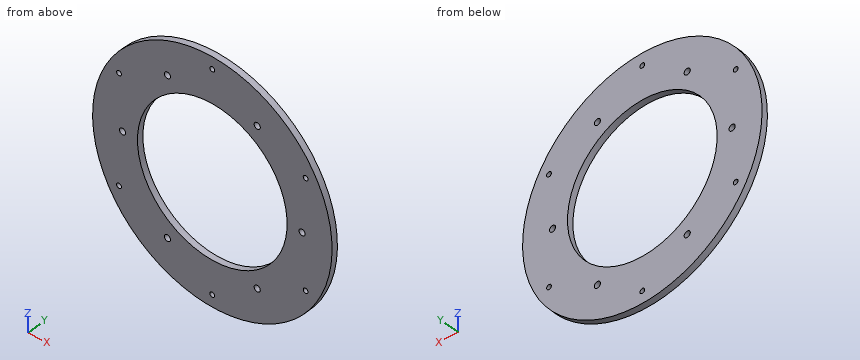
from build123d import *

# Parameters (mm, degrees)
SKETCH_1_R      = 80
SKETCH_1_R_2    = 50
SKETCH_1_R_3    = 2.05
EXTRUDE_1_DEPTH = 4
EXTRUDE_START   = -4
SKETCH_2_R      = 2.05
SKETCH_2_R_2    = 1.6
EXTRUDE_2_DEPTH = 4


with BuildPart() as part:
    # 草图1 → 凸台-拉伸1 (new body)
    with BuildSketch(Plane(origin=(0, 0, 0), x_dir=(1, 0, 0), z_dir=(0, 1, 0))):
        with Locations(Location((0, 0, 0), (0, 0, 270))):
            Circle(SKETCH_1_R)
        with Locations(Location((0, 0, 0), (0, 0, 270))):
            Circle(SKETCH_1_R_2, mode=Mode.SUBTRACT)
        with Locations(Location((60, 0, 0), (0, 0, 270))):
            Circle(SKETCH_1_R_3, mode=Mode.SUBTRACT)
        with Locations(Location((30, -51.961524227, 0), (0, 0, 270))):
            Circle(SKETCH_1_R_3, mode=Mode.SUBTRACT)
        with Locations(Location((-30, -51.961524227, 0), (0, 0, 270))):
            Circle(SKETCH_1_R_3, mode=Mode.SUBTRACT)
        with Locations(Location((-60, 0, 0), (0, 0, 270))):
            Circle(SKETCH_1_R_3, mode=Mode.SUBTRACT)
        with Locations(Location((-30, 51.961524227, 0), (0, 0, 270))):
            Circle(SKETCH_1_R_3, mode=Mode.SUBTRACT)
        with Locations(Location((30, 51.961524227, 0), (0, 0, 270))):
            Circle(SKETCH_1_R_3, mode=Mode.SUBTRACT)
        with Locations(Location((-62.353829072, 36, 0), (0, 0, 270))):
            Circle(SKETCH_1_R_3, mode=Mode.SUBTRACT)
        with Locations(Location((0, 72, 0), (0, 0, 270))):
            Circle(SKETCH_1_R_3, mode=Mode.SUBTRACT)
        with Locations(Location((62.353829072, 36, 0), (0, 0, 270))):
            Circle(SKETCH_1_R_3, mode=Mode.SUBTRACT)
        with Locations(Location((62.353829072, -36, 0), (0, 0, 270))):
            Circle(SKETCH_1_R_3, mode=Mode.SUBTRACT)
        with Locations(Location((0, -72, 0), (0, 0, 270))):
            Circle(SKETCH_1_R_3, mode=Mode.SUBTRACT)
        with Locations(Location((-62.353829072, -36, 0), (0, 0, 270))):
            Circle(SKETCH_1_R_3, mode=Mode.SUBTRACT)
    extrude(amount=EXTRUDE_1_DEPTH)

    # 草图2 → 凸台-拉伸2 (add)
    # profile 1 of 6: a face of its own
    with BuildSketch(Plane(origin=(0, 4, 0), x_dir=(1, 0, 0), z_dir=(0, 1, 0)).offset(EXTRUDE_START)):
        with Locations((62.353829072, 36)):
            Circle(SKETCH_2_R)
        with Locations(Location((62.353829072, 36, 0), (0, 0, 270))):
            Circle(SKETCH_2_R_2, mode=Mode.SUBTRACT)
    # profile 2 of 6: a face of its own
    with BuildSketch(Plane(origin=(0, 4, 0), x_dir=(1, 0, 0), z_dir=(0, 1, 0)).offset(EXTRUDE_START)):
        with Locations((62.353829072, -36)):
            Circle(SKETCH_2_R)
        with Locations(Location((62.353829072, -36, 0), (0, 0, 270))):
            Circle(SKETCH_2_R_2, mode=Mode.SUBTRACT)
    # profile 3 of 6: a face of its own
    with BuildSketch(Plane(origin=(0, 4, 0), x_dir=(1, 0, 0), z_dir=(0, 1, 0)).offset(EXTRUDE_START)):
        with Locations((0, -72)):
            Circle(SKETCH_2_R)
        with Locations(Location((0, -72, 0), (0, 0, 270))):
            Circle(SKETCH_2_R_2, mode=Mode.SUBTRACT)
    # profile 4 of 6: a face of its own
    with BuildSketch(Plane(origin=(0, 4, 0), x_dir=(1, 0, 0), z_dir=(0, 1, 0)).offset(EXTRUDE_START)):
        with Locations((-62.353829072, -36)):
            Circle(SKETCH_2_R)
        with Locations(Location((-62.353829072, -36, 0), (0, 0, 270))):
            Circle(SKETCH_2_R_2, mode=Mode.SUBTRACT)
    # profile 5 of 6: a face of its own
    with BuildSketch(Plane(origin=(0, 4, 0), x_dir=(1, 0, 0), z_dir=(0, 1, 0)).offset(EXTRUDE_START)):
        with Locations((-62.353829072, 36)):
            Circle(SKETCH_2_R)
        with Locations(Location((-62.353829072, 36, 0), (0, 0, 270))):
            Circle(SKETCH_2_R_2, mode=Mode.SUBTRACT)
    # profile 6 of 6: a face of its own
    with BuildSketch(Plane(origin=(0, 4, 0), x_dir=(1, 0, 0), z_dir=(0, 1, 0)).offset(EXTRUDE_START)):
        with Locations((0, 72)):
            Circle(SKETCH_2_R)
        with Locations(Location((0, 72, 0), (0, 0, 270))):
            Circle(SKETCH_2_R_2, mode=Mode.SUBTRACT)
    extrude(amount=EXTRUDE_2_DEPTH)


solid = part.part
Read the model definition and answer for the solid it produces. Units are mm, in the model's axes. Give positions to 0.01 mm unless a question says otherwise; leave off trailing zeros. Write each loop counter-clockwise with the first axis right and the second up, starting at its lowest first coordinate (ties: lowest second). Pieces come first, ordered by that corner, then holes. Notation, with made-up numbers: (5, 63) - (30, 63) arc R15 ccw to (30, 75) - close; hole circle Ø3 at (-5, -23.75). An arc over 180 degrees is marked (long way). Answer in a Markdown table with one row per item. Add a question column.
Item 1: A flat-ended cylindrical pin translates along its axis: P1, Ø1, axis at y = 2, z = -17, coming from the -X side. Find the tip coordinate at first contact, or state that the pin passes through.
Item 2: Section D-D, the plane z = -64 is taken. Write down the section's boundary in (x, y).
Item 3: Section B-B, the plane y = 0.9 is taken. Count the separate pieces of the cut face and the enclosed holes in it, and give its area (3 significant figures).
Item 4: Section A-A, the plane x = -37.5 is taken. Write down the section's boundary in (y, z), and give its area (3 significant figures).
Item 5: Find the intervals of material crossed by L1, parallel to X at y = 2.3, z = 0; L2, parallel to X at y = 2.15, z = -35; L3, parallel to X at y = 0.75, z = 51.5, in increasing order.
Item 6: Section C-C, the plane x = 30 is taken. Write down the section's boundary in (y, z), and give its area (3 significant figures).
Recorded:
| question | item | result |
|---|---|---|
| 1 | P1 | stops at x = -78.28 |
| 2 | outline | (-48, 0) - (48, 0) - (48, 4) - (-48, 4) - close |
| 3 | separate pieces | 1 |
| 3 | enclosed holes | 13 |
| 3 | area | 12,100 mm2 |
| 4 | outline | (0, -70.67) - (4, -70.67) - (4, -33.07) - (0, -33.07) - close; (0, 33.07) - (4, 33.07) - (4, 70.67) - (0, 70.67) - close |
| 4 | area | 301 mm2 |
| 5 | L1 | x = -80 to -62.05, -57.95 to -50, 50 to 57.95, 62.05 to 80 |
| 5 | L2 | x = -71.94 to -63.6, -61.1 to -35.71, 35.71 to 61.1, 63.6 to 71.94 |
| 5 | L3 | x = -61.22 to -32, -28 to 28, 32 to 61.22 |
| 6 | outline | (0, -74.16) - (4, -74.16) - (4, -54.01) - (0, -54.01) - close; (0, -49.91) - (4, -49.91) - (4, -40) - (0, -40) - close; (0, 40) - (4, 40) - (4, 49.91) - (0, 49.91) - close; (0, 54.01) - (4, 54.01) - (4, 74.16) - (0, 74.16) - close |
| 6 | area | 240 mm2 |
